Autodesk Inventor part; units mm, degrees
ref_plane "YZ-Ebene" through (0, 0, 0) normal (1, 0, 0) x (0, 1, 0)
ref_plane "XZ-Ebene" through (0, 0, 0) normal (0, 1, 0) x (-1, 0, 0)
ref_plane "XY-Ebene" through (0, 0, 0) normal (0, 0, 1) x (1, 0, 0)
sketch "Skizze1" plane through (0, 0, 0) normal (0, 0, 1) x (1, 0, 0)
  line L0 (-17.5, 0) -> (-17.5, 29)
  line L1 (-17.5, 29) -> (17.5, 29)
  line L2 (17.5, 29) -> (17.5, 0)
  line L3 (17.5, 0) -> (9, 0)
  line L4 (9, 0) -> (9, -3)
  line L5 (9, -3) -> (-9, -3)
  line L6 (-9, -3) -> (-9, 0)
  line L7 (-9, 0) -> (-17.5, 0)
  point P0 (0, 0)
  point P1 (0, -3)
  point P2 (0, 29)
  point P3 (13.25, 0)
  dimension "d0" = 18
  dimension "d1" = 35
  dimension "d2" = 29
  dimension "d3" = 3
extrude "Extrusion1" add sketch "Skizze1" along normal mid plane 6
sketch "Skizze2" plane through (0, 0, 3) normal (0, 0, 1) x (1, 0, 0)
  line L0 (-11.5, 25) -> (11.5, 25)
  line L1 (11.5, 25) -> (11.5, 2)
  line L2 (11.5, 2) -> (-11.5, 2)
  line L3 (-11.5, 2) -> (-11.5, 25)
  line L4 (-11.5, 25) -> (11.5, 2) construction
  line L5 (11.5, 25) -> (-11.5, 2) construction
  line L6 (-9, -3) -> (9, -3)
  point P0 (0, 0)
  point P1 (0, 13.5)
  point P2 (0, 2)
  dimension "d27" = 16.5
  dimension "d28" = 23
extrude "Extrusion2" cut sketch "Skizze2" against normal blind 4
fillet "Rundung1" radius 5 6 edges at (-17.5, 29, 0) (17.5, 29, 0) (-11.5, 25, 1) (11.5, 25, 1) (11.5, 2, 1) (-11.5, 2, 1)
sketch "Skizze3" plane through (0, 0, -1) normal (0, 0, 1) x (1, 0, 0)
  circle A0 centre (0, 13.5) radius 6.5
  line L0 (-9, -3) -> (9, -3) construction
  line L1 (9, -3) -> (-9, -3) construction
  point P0 (0, 0)
  dimension "d12" = 13
  dimension "d13" = 16.5
extrude "Extrusion3" cut sketch "Skizze3" against normal through all
sketch "Skizze4" plane through (9, 0, 3) normal (0, -1, 0) x (1, 0, 0)
  line L0 (-22.9, -3) -> (-9, -3) construction
  line L1 (-9, -3) -> (4.9, -3) construction
  dimension "d19" = 27.8
hole "Bohrung1" at (-13.9, 0, 0) at (13.9, 0, 0) direction (0, 1, 0) diameter 3.8 depth 8 tip angle 118
sketch "Skizze5" plane through (0, 0, -3) normal (0, 0, -1) x (-1, 0, 0)
  line L0 (-9, -3) -> (-9, 0)
  line L1 (-9, 0) -> (9, 0)
  line L2 (9, 0) -> (9, 5)
  line L3 (9, 5) -> (-9, 5)
  line L4 (-9, 5) -> (-9, 0)
  point P0 (0, 0)
  dimension "d29" = 5
extrude "Extrusion4" add sketch "Skizze5" along normal blind 5
fillet "Rundung2" radius 10.75 2 edges at (9, 2.5, -3) (-9, 2.5, -3)
sketch "Skizze6" plane through (-12.5, 29, -3) normal (0, 1, 0) x (1, 0, 0)
  point P0 (12.5, -3)
hole "Bohrung2" at (0, 29, 0) direction (0, -1, 0) diameter 3.8 depth 4
properties part number "Endcap" material "ABS-Kunststoff"
Can you work these out from the model? Positions are in its coordinate system, mm. A direction names the side the tool comes from. Coordinates: 2 decimals unless noted, no trailing zeros. Loops run counter-clockwise (first coordinate to the right, second up) from the corner with the lowest first, then second, coordinate; pieces in that order, holes last.
1) Which directions (+Z, -Z, +X, -X, +Y, -Y) give clear straight access to the entire face, cutting with the end or side of a thin tool? Please do faces 4 (the flat face through (-11.5, 13, 1)), 5 (the flat face through (0, 25, -1.4)), 6 (the flat face through (9, -1, 0)), 7 (the flat face through (4, 20, -3)).
2) Imagine slicing it at C-C on y = 4. List the corners of the cut face in (x, z) for me.
3) Imagine slicing it at D-D on x = 4.5. List the corners of the cut face in (y, z) for me, plus the area to 3 significant figures.
4) Imagine slicing it at B-B on x = 0. List the corners of the cut face in (y, z) for me.
5) Thinking about a two-plate mould opening in X: for faces 1 (the flat face through (17.5, 12, 0)), 2 (the cylindrical face through (-0.846, 19.945, -1.986)), 3 (the flat face through (-9, -2, 0)), which applies, pulls with the +X half, pulls with the -X half, needs draft (parallel to the pull), parting line crosses it, or undercut?
6) Imagine slicing it at A-A on y = 13.5. List the corners of the cut face in (x, z) for me, plus the area to 3 significant figures.
7) For pin 1 (12 mm diameter, centred on x = 5, y = 13.5, fed in from -Z); pin 2 (2.5 mm diameter, centred on y = -2, z = -1.5, fed in from +X); pin 3 (10.5 mm diameter, centred on x = 0, y = 13.5, fed in from +Z); pin 4 (6 mm diameter, centred on x = 13.9, z = 0, fed in from -Y), each with a flat end and sliding along its axis, tell me the tip position at first contact or that it passes through.
8) I need wall thicknesses on probe 1 along Y at (x, z) = (0, -1.6); probe 2 along Y at (x, z) = (-2.5, 0.5); probe 3 along Z at (x, y) = (-1, 2.5). Which ranges of each line are inside material? Lowest first, please.
Completed:
1. face 4: +Z
1. face 5: +Y
1. face 6: +Z, -Z, +X, -Y
1. face 7: -Z, +X, -X, +Y
2. outline: (-17.5, -3) arc R10.75 cw to (-9, -8) - (9, -8) arc R10.75 cw to (17.5, -3) - (17.5, 3) - (10.5, 3) - (10.5, -1) - (-10.5, -1) - (-10.5, 3) - (-17.5, 3) - close; hole circle Ø3.8 at (-13.9, 0); hole circle Ø3.8 at (13.9, 0)
3. outline: (-3, -3) - (0, -3) - (0, -8) - (5, -8) - (5, -3) - (8.81, -3) - (8.81, -1) - (2, -1) - (2, 3) - (-3, 3) - close; (18.19, -3) - (29, -3) - (29, 3) - (25, 3) - (25, -1) - (18.19, -1) - close
3. area: 106 mm2
4. outline: (-3, -3) - (0, -3) - (0, -8) - (5, -8) - (5, -3) - (7, -3) - (7, -1) - (2, -1) - (2, 3) - (-3, 3) - close; (20, -3) - (29, -3) - (29, -1.9) - (25, -1.9) - (25, -1) - (20, -1) - close; (25, 1.9) - (29, 1.9) - (29, 3) - (25, 3) - close
5. face 1: pulls with the +X half
5. face 2: undercut
5. face 3: pulls with the -X half
6. outline: (-17.5, -3) - (-6.5, -3) - (-6.5, -1) - (-11.5, -1) - (-11.5, 3) - (-17.5, 3) - close; (6.5, -3) - (17.5, -3) - (17.5, 3) - (11.5, 3) - (11.5, -1) - (6.5, -1) - close
6. area: 92.0 mm2
7. pin 1: stops at z = -3
7. pin 2: stops at x = 9
7. pin 3: passes through
7. pin 4: stops at y = 0
8. probe 1: y = -3 to 7, 20 to 25
8. probe 2: y = -3 to 2, 25 to 29
8. probe 3: z = -8 to -1
